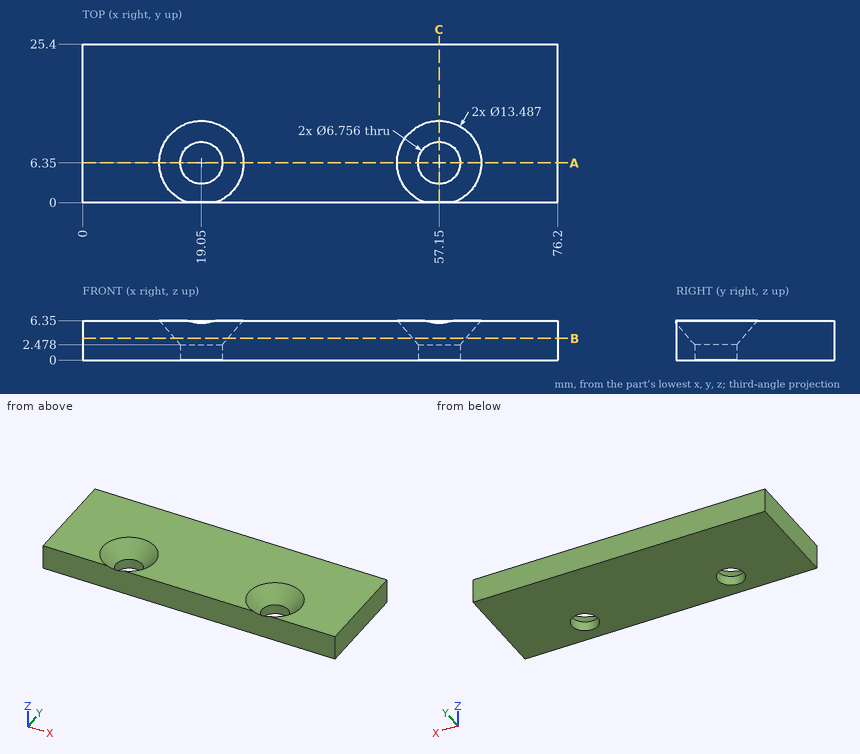
Job drawing, mm, ordinate dimensions from the low corner. One solid piece. Give positions to 0.01 mm unless a question says otherwise; leave off trailing zeros. Write each loop counter-clockwise with the first axis right and the second up, starting at its lowest first coordinate (ties: lowest second). Pieces come first, ordered by that corner, then holes. Notation, with made-up numbers: (-20, -11) - (18, -11) arc R16 ccw to (18, 0) - close; hole circle Ø3 at (-3.5, 24). An arc over 180 degrees is marked (long way). Answer as CSV lines item,"result".
1. Pin check, flat tips, straight feed: pin 1 (5 mm diameter, centred on x = 57.5, y = 9, fed in from -Z); pin 2 (8 mm diameter, centred on x = 19.05, y = 6.35, fed in from +Z) (1 decimal). Stop position of each tip, or through.
Responses:
pin 1,"stops at z = 0"
pin 2,"stops at z = 3.2"
2. Band-saw the part on A-A (y = 6.35). Write the cut outline in (x, z).
Responses:
outline,"(0, 0) - (15.67, 0) - (15.67, 2.48) - (12.31, 6.35) - (0, 6.35) - close; (22.43, 0) - (53.77, 0) - (53.77, 2.48) - (50.41, 6.35) - (25.79, 6.35) - (22.43, 2.48) - close; (60.53, 0) - (76.2, 0) - (76.2, 6.35) - (63.89, 6.35) - (60.53, 2.48) - close"
3. Band-saw the part on B-B (z = 3.5). Write the cut outline in (x, y), and give its area (3 significant figures).
Responses:
outline,"(0, 0) - (76.2, 0) - (76.2, 25.4) - (0, 25.4) - close; hole circle Ø8.53 at (19.05, 6.35); hole circle Ø8.53 at (57.15, 6.35)"
area,"1,820 mm2"
4. Band-saw the part on C-C (x = 57.15). Write the cut outline in (y, z), and give its area (3 significant figures).
Responses:
outline,"(0, 0) - (2.97, 0) - (2.97, 2.48) - (0, 5.9) - close; (9.73, 0) - (25.4, 0) - (25.4, 6.35) - (13.09, 6.35) - (9.73, 2.48) - close"
area,"105 mm2"
5. Drill centre lines: L1, parallel to Y at x = 19.05, z = 1.45; L2, parallel to X at y = 4.5, z = 5.75; L3, parallel to Y at x = 57, z = 3.5 (1 decimal). Where is each one in solid material? Low to high. Write a range as [from, to].
Responses:
L1,"y = [0, 2.97], [9.73, 25.4]"
L2,"x = [0, 13.11], [24.99, 51.21], [63.09, 76.2]"
L3,"y = [0, 2.1], [10.6, 25.4]"
